Drawing for the job (mm, zero at the part's lowest x, y, z). A direction names the side the tool comes from. Coordinates: 2 decimals unless noted, no trailing zeros. Write each loop counter-clockwise with the first axis right and the second up, starting at its lowest first coordinate (ties: lowest second). Pieces come first, ordered by that corner, then holes. Notation, with made-up numbers: M 39,78 L 92,78 A20 ccw 92,93 Z; hole C -17.75,79.25 d8. An arc over 180 degrees is marked long. Use CSV: the item, a comma, the result in double quotes. Start each with the question number.
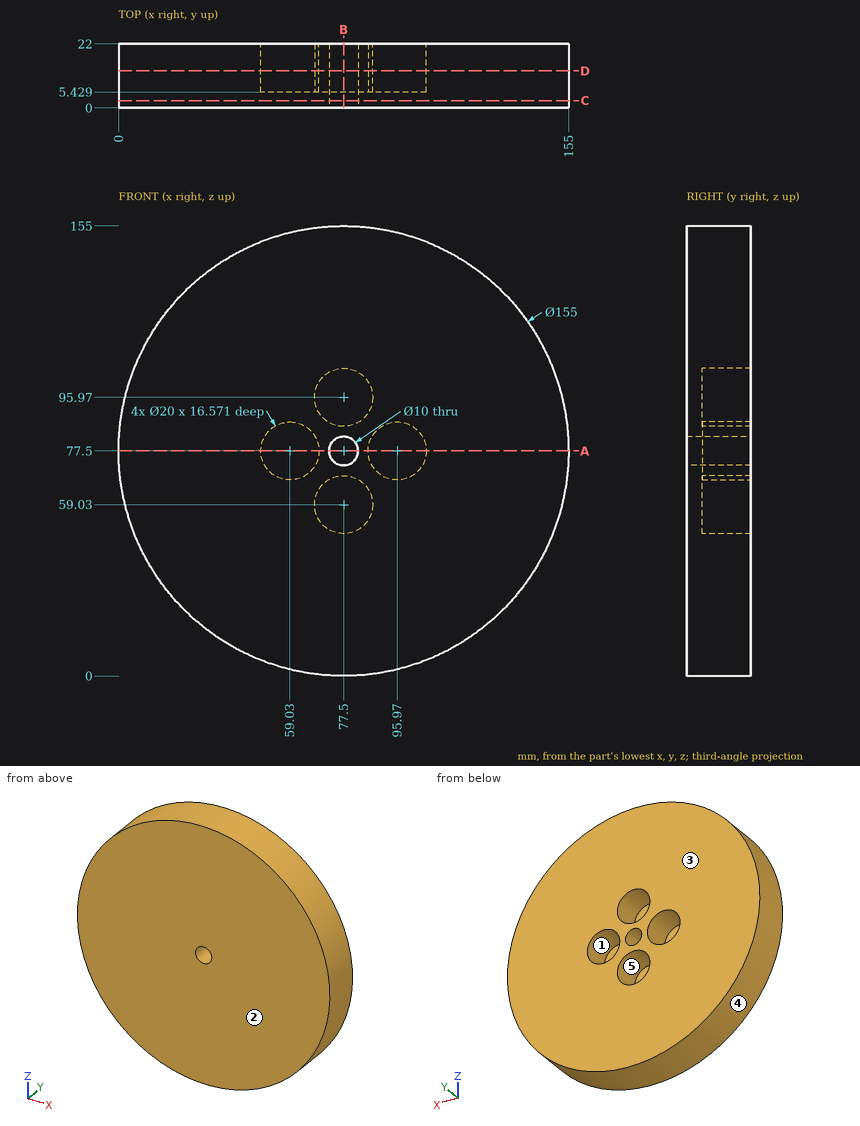
1) Drop flat-ended pins along their axis: P1, Ø6, axis at x = 43.5, y = 9, coming from the +Z side; P2, Ø12, axis at x = 99.5, y = 8, coming from the -Z side; P3, Ø12, axis at y = 5.5, z = 63.5, coming from the +X side. Give the stop position or say it passes through.
2) Tool access for the marked faces 1 and 2: list every direction of +Z, -Z, +X, -X, +Y, -Y with a clear straight run to the whole face (end or side of a thin tool).
3) Band-saw the part on D-D on y = 12.75. List the corners of the cut face in (x, z), then the cut area to 3 significant figures.
4) Band-saw the part on A-A on z = 77.5. List the corners of the cut face in (x, y).
5) Band-saw the part on B-B on x = 77.5. List the corners of the cut face in (y, z).
6) Two-plate mould, pull along X, no slides. Class the marked faces 3, 4 and 5: pulls with the +X half, pulls with the -X half, needs draft (parallel to the pull), parting line crosses it, or undercut.
7) Band-saw the part on C-C on y = 2.5. List the corners of the cut face in (x, z).
8) Wall check: L1, parallel to X at y = 10.25, z = 77.5; L2, parallel to X at y = 14, z = 75.5; L3, parallel to Z at x = 73, y = 7. Give the ranges that are in metal, low to high. Write a range as [from, to].
Findings below:
1,P1,"stops at z = 148.53"
1,P2,"stops at z = 1.67"
1,P3,"stops at x = 154.59"
2,face 1,"+Y"
2,face 2,"+Z, -Z, +X, -X, -Y"
3,outline,"C 77.5,77.5 d155; hole C 59.03,77.5 d20; hole C 77.5,59.03 d20; hole C 77.5,95.97 d20; hole C 77.5,77.5 d10; hole C 95.97,77.5 d20"
3,area,"17,500 mm2"
4,outline,"M 0,0 L 72.5,0 L 72.5,22 L 69.03,22 L 69.03,5.43 L 49.03,5.43 L 49.03,22 L 0,22 Z; M 82.5,0 L 155,0 L 155,22 L 105.97,22 L 105.97,5.43 L 85.97,5.43 L 85.97,22 L 82.5,22 Z"
5,outline,"M 0,0 L 22,0 L 22,49.03 L 5.43,49.03 L 5.43,69.03 L 22,69.03 L 22,72.5 L 0,72.5 Z; M 0,82.5 L 22,82.5 L 22,85.97 L 5.43,85.97 L 5.43,105.97 L 22,105.97 L 22,155 L 0,155 Z"
6,face 3,"needs draft"
6,face 4,"parting line crosses it"
6,face 5,"undercut"
7,outline,"C 77.5,77.5 d155; hole C 77.5,77.5 d10"
8,L1,"x = [0, 49.03], [69.03, 72.5], [82.5, 85.97], [105.97, 155]"
8,L2,"x = [0.03, 49.23], [68.83, 72.92], [82.08, 86.17], [105.77, 154.97]"
8,L3,"z = [0.13, 50.1], [67.96, 75.32], [79.68, 87.04], [104.9, 154.87]"
